```python
from build123d import *

# Parameters (mm, degrees)
SKETCH_2_R          = 62.5
EXTRUDE_1_DEPTH     = 30
FILLET_1_R          = 10
SKETCH_3_R          = 8
CUT_EXTRUDE_1_DEPTH = 31


with BuildPart() as part:
    # 草图2 → 凸台-拉伸1 (new body)
    with BuildSketch(Plane.XY):
        Circle(SKETCH_2_R)
    extrude(amount=EXTRUDE_1_DEPTH)

    # 圆角1
    fillet_1_edges = [part.edges().sort_by_distance(p)[0] for p in [
        (-62.5, 0, 0),
        (-62.5, 0, 30),
    ]]
    fillet(fillet_1_edges, radius=FILLET_1_R)

    # 草图3 → 切除-拉伸1 (cut, through all)
    with BuildSketch(Plane(origin=(0, 0, 0), x_dir=(-1, 0, 0), z_dir=(0, 0, -1))):
        Circle(SKETCH_3_R)
    extrude(amount=-CUT_EXTRUDE_1_DEPTH, mode=Mode.SUBTRACT)


solid = part.part
```
The model under review builds one solid part; all positions refer to its coordinate system, in mm. Round coordinates to 2 decimals unless told otherwise and drop trailing zeros. Loops run counter-clockwise (first coordinate to the right, second up) from the corner with the lowest first, then second, coordinate; pieces in that order, holes last. Notation, with made-up numbers: M 1,-28.5 L 57,-28.5 A5 ccw 57,-24.5 Z; hole C 80.25,-7.75 d7. An arc over 180 degrees is marked long. Write item = value, one per line.
Item 1: Insertion check: P1, Ø10, axis at x = -30, z = 17.5, coming from the -Y side; P2, Ø12, axis at y = 41.5, z = 7.5, coming from the -X side; P3, Ø1.5, axis at y = 14.5, z = 4.5, coming from the -X side. Each pin has a flat end and moves straight along its axis. Give the tip position at first contact, or say it passes through.
Return value:
P1 = -57.28
P2 = -51.25
P3 = -59.6
Item 2: Take a section at A-A on y = 0. Write out the cut boundary in (x, z), then the cut area to 3 significant figures.
Return value:
outline = M -62.5,10 A10 ccw -52.5,0 L -8,0 L -8,30 L -52.5,30 A10 ccw -62.5,20 Z; M 8,0 L 52.5,0 A10 ccw 62.5,10 L 62.5,20 A10 ccw 52.5,30 L 8,30 Z
area = 3,180 mm2
Item 3: Take a section at C-C on z = 26. Write out the cut boundary in (x, y), then the cut area to 3 significant figures.
Return value:
outline = C 0,0 d121; hole C 0,0 d16
area = 11,300 mm2
Item 4: For line 1 (Y direction, x = 0, z = 14.25); line 2 (Y direction, x = 0, z = 6.5); line 3 (X direction, y = -2, z = 28.5), list the stretches that pass through material, from the lowest coordinate up. Write a range as [from, to].
Return value:
line_1 = [-62.5, -8], [8, 62.5]
line_2 = [-61.87, -8], [8, 61.87]
line_3 = [-57.73, -7.75], [7.75, 57.73]
Item 5: Take a section at D-D on z = 2.75. Write out the cut boundary in (x, y), then the cut area to 3 significant figures.
Return value:
outline = C 0,0 d118.77; hole C 0,0 d16
area = 10,900 mm2
Item 6: The part is to be moulded in two halves that separate along Y. For faces 1 (the cylindrical face through (1.73, -7.81, 14.79)), 2 (the cylindrical face through (-62.44, 2.75, 14.93)), 3 (the flat face through (-1, -11, 0)), say which applies: released by +Y, released by -Y, zero draft, split by the parting line, or undercut.
Return value:
face_1 = undercut
face_2 = split by the parting line
face_3 = zero draft
